from build123d import *

# Parameters (mm, degrees)
SKETCH1_W               = 96.012
SKETCH1_H               = 15.875
BASE_EXTRUDE_DEPTH      = 7.9375
CUT_EXTRUDE1_DEPTH      = 98.638740648
FILLET5_R               = 0.635
FILLET6_R               = 3.81
FILLET7_R               = 3.175
FILLET8_R               = 6.35
FILLET9_R               = 6.35
FILLET10_R              = 6.35
BOSS_EXTRUDE3_START     = -6.35
BOSS_EXTRUDE3_DEPTH     = 6.35
FILLET11_R              = 3.81
SKETCH7_R               = 2.54
CUT_EXTRUDE5_DEPTH      = 99.512406834
CUT_EXTRUDE6_DEPTH      = 99.485470295
CUT_EXTRUDE6_DEPTH_BACK = 99.485470295
SKETCH8_W               = 56.651025612
SKETCH8_H               = 0.0254
FILLET12_R              = 3.81
FILLET13_R              = 3.81


with BuildPart() as part:
    # Sketch1 → Base-Extrude (new, symmetric)
    with BuildSketch(Plane.XY):
        with Locations((48.006, 7.9375)):
            Rectangle(SKETCH1_W, SKETCH1_H)
    extrude(amount=BASE_EXTRUDE_DEPTH, both=True)

    # Sketch3 → Cut-Extrude1 (cut, through all)
    with BuildSketch(Plane(origin=(0, 15.875, 0), x_dir=(-1, 0, 0), z_dir=(0, 1, 0))):
        Polygon((-53.213, -4.7625), (-92.837, -4.7625), (-92.837, 4.7625), (-53.213, 4.7625), (-48.4505, 0), align=None)
        Polygon((2.11806403, -3.175), (-47.135371939, -3.175), (-55.848364541, -11.887992602), (2.11806403, -11.887992602), align=None)
        Polygon((2.11806403, 3.175), (-47.135371939, 3.175), (-55.848364541, 11.887992602), (2.11806403, 11.887992602), align=None)
    extrude(amount=-CUT_EXTRUDE1_DEPTH, mode=Mode.SUBTRACT)

    # Fillet5
    fillet5_edges = [part.edges().sort_by_distance(p)[0] for p in [
        (53.213, 7.9375, -4.7625),
        (53.213, 7.9375, 4.7625),
        (47.135371939, 7.9375, 3.175),
        (47.135371939, 7.9375, -3.175),
    ]]
    fillet(fillet5_edges, radius=FILLET5_R)

    # Fillet6
    fillet6_edges = [part.edges().sort_by_distance(p)[0] for p in [
        (51.897871939, 7.9375, 7.9375),
        (51.897871939, 7.9375, -7.9375),
    ]]
    fillet(fillet6_edges, radius=FILLET6_R)

    # Fillet7
    fillet7_edges = [part.edges().sort_by_distance(p)[0] for p in [
        (92.837, 7.9375, -4.7625),
        (92.837, 7.9375, 4.7625),
    ]]
    fillet(fillet7_edges, radius=FILLET7_R)

    # Fillet8
    fillet8_edges = [part.edges().sort_by_distance(p)[0] for p in [
        (96.012, 7.9375, 7.9375),
        (96.012, 7.9375, -7.9375),
    ]]
    fillet(fillet8_edges, radius=FILLET8_R)

    # Fillet9
    fillet9_edges = [part.edges().sort_by_distance(p)[0] for p in [
        (0, 15.875, 0),
    ]]
    fillet(fillet9_edges, radius=FILLET9_R)

    # Fillet10
    fillet10_edges = [part.edges().sort_by_distance(p)[0] for p in [
        (0, 0, 0),
    ]]
    fillet(fillet10_edges, radius=FILLET10_R)

    # Sketch6 → Boss-Extrude3 (add)
    with BuildSketch(Plane.XY.offset(3.175).offset(BOSS_EXTRUDE3_START)):
        with BuildLine():
            Line((5.564108911, 15.826180461), (30.825163366, 18.976770691))
            ThreePointArc((30.825163366, 18.976770691), (39.943880119, 14.786551928), (40.249024971, 4.755808431))
            ThreePointArc((40.249024971, 4.755808431), (36.72434383, -2.446073762), (28.949130797, -4.404784191))
            Line((28.949130797, -4.404784191), (5.165376283, 0.111477206))
            ThreePointArc((5.165376283, 0.111477206), (1.458943846, 2.300300048), (0, 6.35))
            Line((0, 6.35), (0, 9.525))
            ThreePointArc((0, 9.525), (1.590120358, 13.728099546), (5.564108911, 15.826180461))
        make_face()
    extrude(amount=BOSS_EXTRUDE3_DEPTH)

    # Fillet11
    fillet11_edges = [part.edges().sort_by_distance(p)[0] for p in [
        (38.862, 0, 0),
        (39.103515829, 15.875, 0),
    ]]
    fillet(fillet11_edges, radius=FILLET11_R)

    # Sketch7 → Cut-Extrude5 (cut, through all)
    with BuildSketch(Plane.XY.offset(3.175)):
        with Locations((6.35, 9.525)):
            Circle(SKETCH7_R)
        with Locations((32.004, 9.525)):
            Circle(SKETCH7_R)
    extrude(amount=-CUT_EXTRUDE5_DEPTH, mode=Mode.SUBTRACT)

    # Sketch8 → Cut-Extrude6 (cut, two sides: drawn at the far end of the back side and taken through both)
    with BuildSketch(Plane(origin=(0, 15.875, 0), x_dir=(-1, 0, 0), z_dir=(0, 1, 0)).offset(-CUT_EXTRUDE6_DEPTH_BACK)):
        with Locations((-25.150512806, 0)):
            Rectangle(SKETCH8_W, SKETCH8_H)
    extrude(amount=CUT_EXTRUDE6_DEPTH + CUT_EXTRUDE6_DEPTH_BACK, mode=Mode.SUBTRACT)

    # Fillet12
    fillet12_edges = [part.edges().sort_by_distance(p)[0] for p in [
        (48.4632, 7.9375, 0.0127),
    ]]
    fillet(fillet12_edges, radius=FILLET12_R)

    # Fillet13
    fillet13_edges = [part.edges().sort_by_distance(p)[0] for p in [
        (48.4632, 7.9375, -0.0127),
    ]]
    fillet(fillet13_edges, radius=FILLET13_R)


solid = part.part
Design review of the part built by this model. Coordinates are the model's own, in mm. A direction names the side the tool comes from. Coordinates: 2 decimals unless noted, no trailing zeros. Loops run counter-clockwise (first coordinate to the right, second up) from the corner with the lowest first, then second, coordinate; pieces in that order, holes last. Notation, with made-up numbers: (-24.5, -36) - (-4.5, -36) arc R17 ccw to (-4.5, -11) - close; hole circle Ø8 at (6.25, -15). An arc over 180 degrees is marked (long way). Use CSV: the item, a comma, the result in double quotes. Start each with the question number.
1. To check wall thickness, follow probe 1 along Z at (x, y) = (81.5, 7.5); probe 2 along X at (y, z) = (5.25, -4.5); probe 3 along X at (y, z) = (0.5, -2). State the ranges of each line that lie inside material, in increasing order.
2. Clearance check with flat-ended pins moving along their axes: pin 1 (4 mm diameter, centred on x = 46.5, z = -0.5, fed in from +Y) (3 decimals); pin 2 (8 mm diameter, centred on x = 42, y = 5, fed in from +Z) (3 decimals); pin 3 (6 mm diameter, centred on x = 25, z = -1, fed in from +Y); pin 4 (4.5 mm diameter, centred on x = 32.004, y = 9.525, fed in from -Z). State where each tip first meets the part, or that it passes through.
3. Add section A-A on x = 83.5. Give the boundary of the cut face in (y, z) (1 decimal).
4. For faces 1 (the flat face through (24, 7, -3.175)), 2 (the flat face through (72, 8, 4.762)), 3 (the flat face through (68, 15.875, -5)), 4 (the flat face through (24, 7, 3.175)), list the 3-axis set-ups (+Z, -Z, +X, -X, +Y, -Y) from which the entire face can be reached by the end or side of a thin tool; tool diameter is ignored.
5. Mouldability with a two-part tool opening along Z and no side actions: class faces 5 (the cylindrical face through (91.93, 7.83, -3.81)), 6 (the cylindrical face through (33.906, -4.026, 1.572)), 7 (the flat face through (71, 8, -4.762)), 8 (the flat face through (71, 8, 7.938)) as released by +Z, released by -Z, zero draft, split by the parting line, or undercut.
6. Add section C-C on x = 35.5. Give the boundary of the cut face in (y, z) (3 decimals), plus the area to 3 significant figures.
Resolved:
1,probe 1,"-7.94 to -4.76, 4.76 to 7.94"
1,probe 2,"48.46 to 52.95, 90.93 to 95.3"
1,probe 3,"3.88 to 50.45, 92.81 to 96"
2,pin 1,"y = 15.875"
2,pin 2,"z = 3.175"
2,pin 3,"y = 18.62"
2,pin 4,"through"
3,outline,"(0, -7.9) - (15.9, -7.9) - (15.9, -4.8) - (0, -4.8) - close; (0, 4.8) - (15.9, 4.8) - (15.9, 7.9) - (0, 7.9) - close"
4,face 1,"-Z, -X, +Y, -Y"
4,face 2,"+Y, -Y"
4,face 3,"+Z, -Z, +X, +Y"
4,face 4,"+Z, -X, +Y, -Y"
5,face 5,"undercut"
5,face 6,"zero draft"
5,face 7,"undercut"
5,face 8,"released by +Z"
6,outline,"(-3.289, -3.175) - (18.385, -3.175) - (18.385, -0.013) - (-3.289, -0.013) - close; (-3.289, 0.013) - (18.385, 0.013) - (18.385, 3.175) - (-3.289, 3.175) - close"
6,area,"137 mm2"
